from build123d import *


with BuildPart() as part:
    # Sketch1 → Revolve1 (revolve)
    with BuildSketch(Plane.XY, mode=Mode.PRIVATE) as revolve1_sk:
        with BuildLine():
            Line((-10, -44.908203932), (-10, -45.908203932))
            ThreePointArc((-10, -45.908203932), (-13.162169665, -49.978471046), (-12, -55))
            Line((-12, -55), (-15, -57))
            Line((-15, -57), (-15, -60))
            Line((-15, -60), (0, -60))
            Line((0, -60), (0, 0))
            ThreePointArc((0, 0), (-8.407551231, -5.788601192), (-6, -15.708203932))
            ThreePointArc((-6, -15.708203932), (-6.8, -17.308203932), (-6, -18.908203932))
            ThreePointArc((-6, -18.908203932), (-5.533425696, -31.030418458), (-8, -42.908203932))
            ThreePointArc((-8, -42.908203932), (-9.414213562, -43.49399037), (-10, -44.908203932))
        make_face()
    revolve(revolve1_sk.sketch.rotate(Axis((0, 67.872071481, 0), (0, -1, 0)), 270), axis=Axis((0, 67.872071481, 0), (0, -1, 0)))


solid = part.part
Build history of the part. All positions in model axes, mm. Round coordinates to 2 decimals unless told otherwise and drop trailing zeros. Write each loop counter-clockwise with the first axis right and the second up, starting at its lowest first coordinate (ties: lowest second). Pieces come first, ordered by that corner, then holes. Notation, with made-up numbers: M -7,44.25 L 25,44.25 A26 cw 25,68.25 Z; hole C 26,-17 d8. An arc over 180 degrees is marked long. Answer as a JSON object with one key per item and string values. Group by question number.
(1) Mould opens along Y. For faces 1 (the cylindrical face through (9.76, -45.42, -2.17)), 2 (the conical face through (-3.661, -55.125, 11.625)), 3 (the flat face through (0, -60, 0)) say: pulls with the +Y half, pulls with the -Y half, needs draft (parallel to the pull), parting line crosses it, or undercut.
(2) Flat gauge pins, fed straight in: pin 1 (1 mm diameter, centred on x = 2, y = -10.5, fed in from +Z); pin 2 (1.5 mm diameter, centred on y = -50, z = 4, fed in from +X); pin 3 (5 mm diameter, centred on x = -1.5, y = -16, fed in from -Z). Where does each tip first touch, or does it go through?
(3) Cut at A-A (z = 0). Give the cut face in (x, y).
(4) Cut at C-C (y = -43.5). Give the cut face in (x, z).
(5) Cut at B-B (x = 0). Give the cut face in (y, z), and give its area (3 significant figures).
(6) Drill centre lines: L1, parallel to Y at x = 10, z = 11; L2, parallel to Z at x = 4.75, y = -5.5; L3, parallel to Z at x = -1.75, y = -23.5. Where is each one in solid material? Low to high.
Responses:
{
 "1": {"face 1": "needs draft", "face 2": "undercut", "face 3": "pulls with the -Y half"},
 "2": {"pin 1": "stops at z = 8.77", "pin 2": "stops at x = 12.8", "pin 3": "stops at z = -7.7"},
 "3": {"outline": "M -15,-60 L 15,-60 L 15,-57 L 12,-55 A6 ccw 10,-45.91 L 10,-44.91 A2 ccw 8,-42.91 A50 cw 6,-18.91 A2 ccw 6,-15.71 A9 ccw long -6,-15.71 A2 ccw -6,-18.91 A50 cw -8,-42.91 A2 ccw -10,-44.91 L -10,-45.91 A6 ccw -12,-55 L -15,-57 Z"},
 "4": {"outline": "C 0,0 d18.84"},
 "5": {"outline": "M -60,-15 L -57,-15 L -55,-12 A6 ccw -45.91,-10 L -44.91,-10 A2 ccw -42.91,-8 A50 cw -18.91,-6 A2 ccw -15.71,-6 A9 ccw long -15.71,6 A2 ccw -18.91,6 A50 cw -42.91,8 A2 ccw -44.91,10 L -45.91,10 A6 ccw -55,12 L -57,15 L -60,15 Z", "area": "997 mm2"},
 "6": {"L1": "y = -60 to -56.91", "L2": "z = -6.8 to 6.8", "L3": "z = -5.19 to 5.19"}
}
